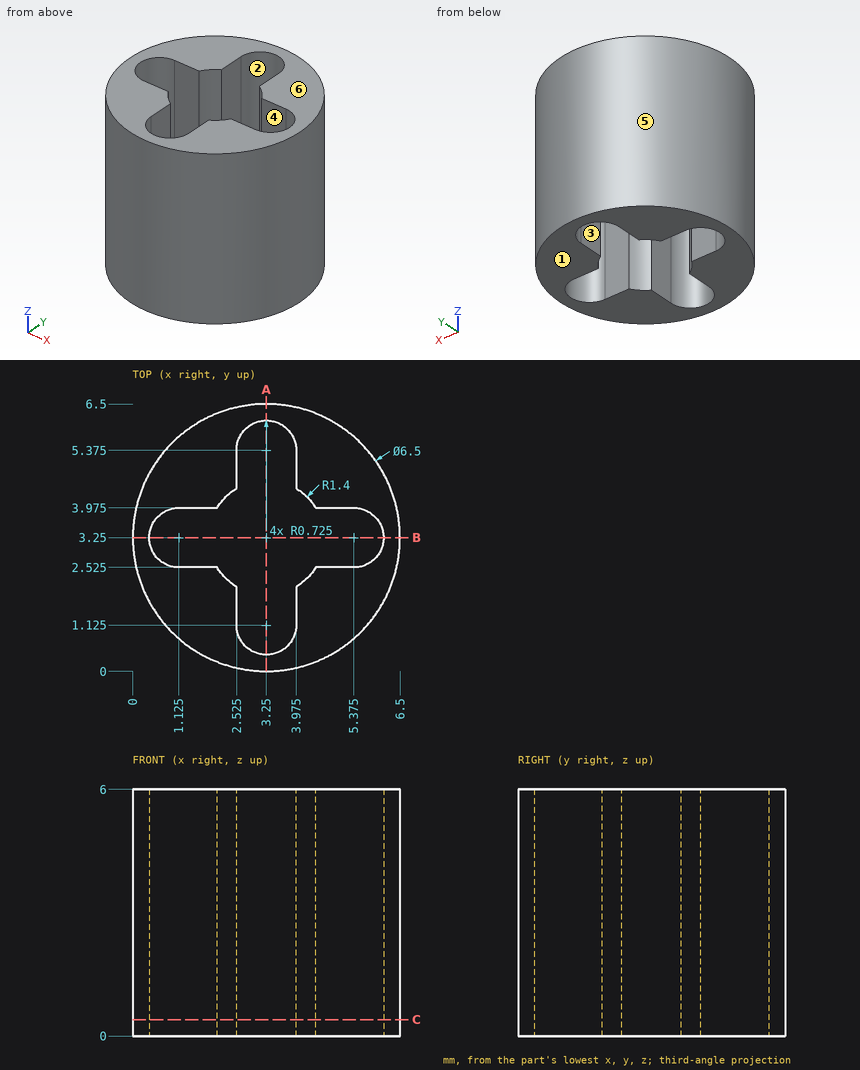
Geometry check sheet. Reference: drawing and pictorial views, mm from the part's lowest x, y, z. A direction names the side the tool comes from. Round coordinates to 2 decimals unless told otherwise and drop trailing zeros. Loops run counter-clockwise (first coordinate to the right, second up) from the corner with the lowest first, then second, coordinate; pieces in that order, holes last. Notation, with made-up numbers: M 9.25,36.5 L 44.25,36.5 A31 ccw 44.25,73.5 Z; hole C -8,-24 d7. An arc over 180 degrees is marked long. Return JSON: item names as keys, results as strings. Group by question number.
(1) Mould release check, pull along Y, two halves, no side actions. Record for the marked faces 3, 4, 5 and 6: pulls with the +Y half, pulls with the -Y half, needs draft (parallel to the pull), parting line crosses it, or undercut.
(2) Section check C-C, the plane z = 0.4. Enter the section's corners in (x, y) (3 decimals), and give its area (3 significant figures).
(3) Go/stop test with flat-tipped pins: pin 1 (0.7 mm diameter, centred on x = 5, z = 4.5, fed in from -Y); pin 2 (1 mm diameter, centred on x = 1.5, z = 3, fed in from +Y); pin 3 (1 mm diameter, centred on x = 2, z = 4, fed in from -Y). Record where each tip stops, or that it passes through.
(4) Section check A-A, the plane x = 3.25. Enter the section's corners in (y, z).
(5) Scan lines: line 1 along Y through (x, z) = (3.25, 1.8); line 2 along X through (y, z) = (4.5, 1.8) (3 decimals); line 3 along X through (y, z) = (3.5, 2.75). Record each from-to range of solid material in increasing order. Write a range as [from, to].
(6) Set-up check for the marked faces 1 and 2: record each of +Z, -Z, +X, -X, +Y, -Y from which the full face is reachable in a straight line by a thin tool's end or side.
Data:
{
 "1": {"face 3": "undercut", "face 4": "undercut", "face 5": "parting line crosses it", "face 6": "needs draft"},
 "2": {"outline": "C 3.25,3.25 d6.5; hole M 1.125,2.525 L 2.052,2.525 A1.4 ccw 2.525,2.052 L 2.525,1.125 A0.725 ccw 3.975,1.125 L 3.975,2.052 A1.4 ccw 4.448,2.525 L 5.375,2.525 A0.725 ccw 5.375,3.975 L 4.448,3.975 A1.4 ccw 3.975,4.448 L 3.975,5.375 A0.725 ccw 2.525,5.375 L 2.525,4.448 A1.4 ccw 2.052,3.975 L 1.125,3.975 A0.725 ccw Z", "area": "19.1 mm²"},
 "3": {"pin 1": "y = 0.32", "pin 2": "y = 6.25", "pin 3": "y = 0.09"},
 "4": {"outline": "M 0,0 L 0.4,0 L 0.4,6 L 0,6 Z; M 6.1,0 L 6.5,0 L 6.5,6 L 6.1,6 Z"},
 "5": {"line 1": "[0, 0.4], [6.1, 6.5]", "line 2": "[0.25, 2.525], [3.975, 6.25]", "line 3": "[0.01, 0.44], [6.06, 6.49]"},
 "6": {"face 1": "-Z, +X, -X, +Y, -Y", "face 2": "+Z, -Z"}
}
